```python
from build123d import *

# Parameters (mm, degrees)
F1_DEPTH = 2
F2_DEPTH = 4
F3_R     = 5
F4_R     = 3


with BuildPart() as f1:
    # F0 (on Top) → F1 (new body)
    with BuildSketch(Plane.XY):
        Polygon((3.6705210805, 7.0790494792), (2.404163056, 7.0790494792), (2.404163056, 5.3348351503), (0, 2.9306720942), (0, 0.5860975944), (3.6705210805, 4.2566186748), align=None)
        Polygon((2.404163056, -5.3348351503), (2.404163056, -7.0790494792), (3.6705210805, -7.0790494792), (3.6705210805, -4.2566186748), (0, -0.5860975944), (0, -2.9306720942), align=None)
        Polygon((0, -5.3348351503), (0, -7.0790494792), (2.404163056, -7.0790494792), (2.404163056, -5.3348351503), (0, -2.9306720942), align=None)
        Polygon((-7.0790494792, 0), (0, -7.0790494792), (0, -5.3348351503), (-5.3348351503, 0), (0, 5.3348351503), (0, 7.0790494792), align=None)
        Polygon((2.404163056, 7.0790494792), (0, 7.0790494792), (0, 5.3348351503), (0, 2.9306720942), (2.404163056, 5.3348351503), align=None)
        Polygon((-5.3348351503, 0), (0, -5.3348351503), (0, -2.9306720942), (-2.9306720942, 0), (0, 2.9306720942), (0, 5.3348351503), align=None)
        Polygon((-2.9306720942, 0), (0, -2.9306720942), (0, -0.5860975944), (-0.5860975944, 0), (0, 0.5860975944), (0, 2.9306720942), align=None)
    extrude(amount=-F1_DEPTH)

    # F0 (on Top) → F2 (join)
    with BuildSketch(Plane.XY):
        Polygon((-7.0790494792, 0), (0, -7.0790494792), (0, -5.3348351503), (-5.3348351503, 0), (0, 5.3348351503), (0, 7.0790494792), align=None)
        Polygon((-2.9306720942, 0), (0, -2.9306720942), (0, -0.5860975944), (-0.5860975944, 0), (0, 0.5860975944), (0, 2.9306720942), align=None)
        Polygon((3.6705210805, 7.0790494792), (2.404163056, 7.0790494792), (2.404163056, 5.3348351503), (0, 2.9306720942), (0, 0.5860975944), (3.6705210805, 4.2566186748), align=None)
        Polygon((2.404163056, -5.3348351503), (2.404163056, -7.0790494792), (3.6705210805, -7.0790494792), (3.6705210805, -4.2566186748), (0, -0.5860975944), (0, -2.9306720942), align=None)
    extrude(amount=F2_DEPTH)

    # F3
    f3_edges = [f1.edges().sort_by_distance(p)[0] for p in [
        (-2.930672, 0, 2),
        (-0.586098, 0, 1),
        (-5.334835, 0, 2),
        (-7.079049, 0, 1),
    ]]
    fillet(f3_edges, radius=F3_R)

    # F4
    f4_edges = [f1.edges().sort_by_distance(p)[0] for p in [
        (2.404163, -5.334835, 2),
        (0, -5.334835, 2),
        (0, 5.334835, 2),
        (2.404163, 5.334835, 2),
    ]]
    fillet(f4_edges, radius=F4_R)


solid = f1.part
```
For this review, take the finished solid that the model builds, in its own axes (mm). A direction names the side the tool comes from. Give positions to 0.01 mm unless a question says otherwise; leave off trailing zeros. Order: outer loops, then holes, each group sorted by start corner. A loop starts at its lowest first (then second) coordinate and runs counter-clockwise, first axis right, second up.
1) Take a section at C-C (x = -3.75). Give the boundary of the cut face in (y, z).
2) Take a section at A-A (x = -2.25). Give the boundary of the cut face in (y, z), then the cut area to 3 significant figures.
3) Take a section at B-B (y = 3.75). Give the boundary of the cut face in (x, z), then the cut area to 3 significant figures.
4) For faces 5 (the face through (2.169, 5.414, 2.028)), 6 (the face through (1.06, -3.99, 1.97)), 7 (the face through (-1, 0, -2)), 8 (the face through (-0.222, 5.445, 2.028)), list the 3-axis set-ups (+Z, -Z, +X, -X, +Y, -Y) from which the entire face can be reached by the end or side of a thin tool; tool diameter is ignored.
5) Insertion check: pin 1 (0.6 mm diameter, centred on y = -7, z = 3, fed in from -X). The pin has a flat end and moves straight along its axis. Give the tip position at first contact, or say it passes through.
6) The part is to be moulded in two halves that separate along X. For faces 1 (the face through (-0.222, -5.445, 2.028)), 2 (the face through (-5.008, -0.055, 0.958)), 3 (the face through (3.671, -6, 1)), 4 (the face through (1, 0, 4)), say which applies: released by +X, released by -X, zero draft, split by the parting line, or undercut.
7) Wall thickness on line 1 (X direction, y = 0, z = 2.75); line 2 (Y direction, x = -0.5, z = -1.5); line 3 (X direction, y = 1.5, z = 2.25): over which ranges is each line inside the solid? List them lowest first.
Derived:
1. outline: (-3.32, -2) - (3.32, -2) - (3.32, 4) - (-3.32, 4) - close
2. outline: (-4.83, -2) - (4.83, -2) - (4.83, 4) - (3.02, 4) - (3.02, 0) - (-3.02, 0) - (-3.02, 4) - (-4.83, 4) - close
2. area: 33.8 mm2
3. outline: (-3.33, -2) - (3.16, -2) - (3.16, 4) - (0.82, 4) - (0.82, 0) - (-1.58, 0) - (-1.58, 4) - (-3.33, 4) - close
3. area: 29.3 mm2
4. face 5: +Z, +Y
4. face 6: +Z, -Y
4. face 7: -Z, +X, -X, +Y, -Y
4. face 8: +Z
5. pin 1: stops at x = -0.38
6. face 1: undercut
6. face 2: released by -X
6. face 3: released by +X
6. face 4: zero draft
7. line 1: x = -5.01 to -3.26, -0.86 to 1.48
7. line 2: y = -6.58 to 6.58
7. line 3: x = -4.78 to -3.03, -0.63 to 1.72
